Autodesk Inventor part; units mm, degrees
ref_plane "YZ Plane" through (0, 0, 0) normal (1, 0, 0) x (0, 1, 0)
ref_plane "XZ Plane" through (0, 0, 0) normal (0, 1, 0) x (-1, 0, 0)
ref_plane "XY Plane" through (0, 0, 0) normal (0, 0, 1) x (1, 0, 0)
sketch "Sketch1" plane through (0, 0, 0) normal (0, 0, 1) x (1, 0, 0)
  line L0 (0, 0) -> (10, 0)
  line L1 (0, 0) -> (-10, 0)
  line L2 (-10, 0) -> (-10, -6.5)
  line L3 (10, 0) -> (10, -6.5)
  line L4 (-10, 0) -> (10, 0)
  line L5 (-10, -20) -> (10, -20)
  line L6 (-10, -6.5) -> (-10, -5)
  line L7 (-6, -5) -> (6, -5)
  line L8 (-6, -15) -> (6, -15)
  line L9 (6, -5) -> (6, -15)
  line L10 (-6, -5) -> (-6, -15)
  line L11 (-10, 0) -> (-10, -6.5)
  line L12 (-10, -13.5) -> (-10, -20)
  line L13 (10, -20) -> (10, -13.5)
  line L14 (10, -6.5) -> (10, 0)
  circle A0 centre (10, -10) radius 1.5
  arc A1 (10, -13.5) -> (10, -6.5) centre (10, -10) ccw
  circle A2 centre (-10, -10) radius 1.5
  arc A3 (-10, -6.5) -> (-10, -13.5) centre (-10, -10) ccw
  dimension "d0" = 10
  dimension "d1" = 10
  dimension "d2" = 20
  dimension "d7" = 3
  dimension "d8" = 7
  dimension "d9" = 3
  dimension "d10" = 7
extrude "Extrusion1" add sketch "Sketch1" along normal blind 2
thread "Thread2"
thread "Thread3"
sketch "Sketch6" plane through (0, 0, 2) normal (0, 0, 1) x (1, 0, 0)
  line L0 (10, 0) -> (-10, 0)
  line L1 (-5, 0) -> (-5, 20)
  line L2 (-5, 0) -> (15, 0) construction
  line L3 (-5, 20) -> (5, 20)
  line L4 (5, 20) -> (5, 0)
  arc A0 (-10, -6.5) -> (-10, -13.5) centre (-10, -10) ccw
  arc A1 (10, -13.5) -> (10, -6.5) centre (10, -10) ccw
  line L5 (-13.5, -10) -> (13.5, -10)
  circle A2 centre (0, 10) radius 2.125
  point P0 (0, 0)
  dimension "d45" = 20
  dimension "d47" = 10
  dimension "d59" = 4.25
extrude "Extrusion7" add sketch "Sketch6" against normal blind 2
properties part number "Time of Flight Attachment 2.0"
CAD build for the part. Positions are in the model's coordinates, mm. A direction names the side the tool comes from. Give positions to 0.01 mm unless a question says otherwise; leave off trailing zeros. Loops run counter-clockwise (first coordinate to the right, second up) from the corner with the lowest first, then second, coordinate; pieces in that order, holes last. Notation, with made-up numbers: M 65,67.25 L 104,67.25 A28 cw 104,99.25 Z; hole C -20.75,85 d10. An arc over 180 degrees is marked long. Use one line per item in the form item = value.
Item 1: Slice it at B-B (y = -10). List the corners of the cut face in (x, z), plus the area to 3 significant figures.
Determined:
outline = M -13.5,0 L -11.5,0 L -11.5,2 L -13.5,2 Z; M -8.5,0 L -6,0 L -6,2 L -8.5,2 Z; M 6,0 L 8.5,0 L 8.5,2 L 6,2 Z; M 11.5,0 L 13.5,0 L 13.5,2 L 11.5,2 Z
area = 18.0 mm2
Item 2: Flat gauge pins, fed straight in: pin 1 (1 mm diameter, centred on y = 15, z = 0.5, fed in from -X); pin 2 (0.6 mm diameter, centred on y = -1.5, z = 1, fed in from +X); pin 3 (1.8 mm diameter, centred on x = 10, y = -10, fed in from +Z); pin 4 (0.6 mm diameter, centred on y = -10.5, z = 0.5, fed in from -X). Where does each tip first touch, or does it go through?
Determined:
pin_1 = -5
pin_2 = 10
pin_3 = through
pin_4 = -13.49
Item 3: Two-plate mould, pull along Y, no slides. Class faces 1 (the face through (0, -5, 1)), 2 (the face through (0, 20, 1)), 3 (the face through (-0.461, 7.926, 1.014)), 4 (the face through (-13.5, -10.1, 1)): pulls with the +Y half, pulls with the -Y half, needs draft (parallel to the pull), parting line crosses it, or undercut.
Determined:
face_1 = undercut
face_2 = pulls with the +Y half
face_3 = undercut
face_4 = parting line crosses it
Item 4: Which spindle directions (+Z, -Z, +X, -X, +Y, -Y) get a long thin tool onto all of the face, cutting with end or side? Do faces 5 (the face through (10, -17, 1)), 6 (the face through (-5, 10, 1)), 7 (the face through (6, -10, 1)). Say none if no direction does.
Determined:
face_5 = +Z, -Z, +X, -Y
face_6 = +Z, -Z, -X, +Y
face_7 = +Z, -Z
Item 5: Slice it at A-A (x = 0). List the corners of the cut face in (y, z) (3 decimals).
Determined:
outline = M -20,0 L -15,0 L -15,2 L -20,2 Z; M -5,0 L 7.875,0 L 7.875,2 L -5,2 Z; M 12.125,0 L 20,0 L 20,2 L 12.125,2 Z
Item 6: Drill centre lines: probe 1 along Y at (x, z) = (0, 1.5) (3 decimals); probe 2 along Y at (x, z) = (-3.25, 1.5); probe 3 along Y at (x, z) = (-0.75, 0.7). Where is each one in solid material? Low to high. Write a range as from..to.
Determined:
probe_1 = -20..-15, -5..7.875, 12.125..20
probe_2 = -20..-15, -5..20
probe_3 = -20..-15, -5..8.01, 11.99..20
Item 7: Slice it at C-C (y = 10). List the corners of the cut face in (x, z) (3 decimals), plus the area to 3 significant figures.
Determined:
outline = M -5,0 L -2.125,0 L -2.125,2 L -5,2 Z; M 2.125,0 L 5,0 L 5,2 L 2.125,2 Z
area = 11.5 mm2
Item 8: Slice it at D-D (z = 1). List the corners of the cut face in (x, y) (3 decimals).
Determined:
outline = M -10,-20 L 10,-20 L 10,-13.5 A3.5 ccw 10,-6.5 L 10,0 L 5,0 L 5,20 L -5,20 L -5,0 L -10,0 L -10,-6.5 A3.5 ccw -10,-13.5 Z; hole C -10,-10 d3; hole M -6,-15 L 6,-15 L 6,-5 L -6,-5 Z; hole C 0,10 d4.25; hole C 10,-10 d3
